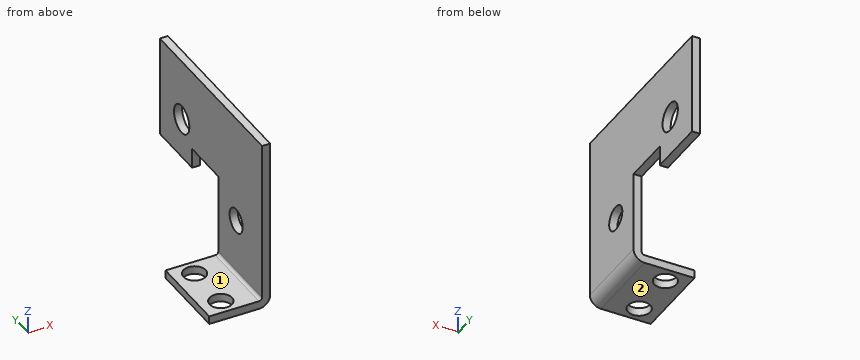
```python
from build123d import *

# Parameters (mm, degrees)
SKETCH_1_W                       = 2
SKETCH_1_H                       = 50
SM_BASE_FLANGE_1_DEPTH           = 35.2
SKETCH_7_W                       = 16.759406963
SKETCH_7_H                       = 59.520719971
CUT_EXTRUDE_2_DEPTH              = 4.8
SKETCH_9_W                       = 8.068883198
SKETCH_9_H                       = 35.697926428
CUT_EXTRUDE_3_DEPTH              = 3.23
SKETCH_6_R                       = 3.5
CUT_EXTRUDE_5_DEPTH              = 10
SKETCH_15_W                      = 15.322876818
SKETCH_15_H                      = 12
CUT_EXTRUDE_7_DEPTH              = 10
SKETCH_18_R                      = 3
CUT_EXTRUDE_8_DEPTH              = 10
SKETCH_19_W                      = 2
SKETCH_19_H                      = 14.77
SKETCH_19_H_2                    = 20
EXTRUDE_1_DEPTH                  = 2.66
SKETCH_20_W                      = 8
SKETCH_20_H                      = 14.77
CUT_EXTRUDE_9_DEPTH              = 8
SKETCH_21_W                      = 2
SKETCH_21_H                      = 20
EXTRUDE_2_DEPTH                  = 9.51
SM_EDGE_FLANGE_1_STRIP_W         = 9.4732
SM_EDGE_FLANGE_1_STRIP_H         = 2
SM_EDGE_FLANGE_1_STRIP_CUT_DEPTH = 20
SM_EDGE_FLANGE_1_DEPTH           = 20
SKETCH_27_R                      = 2.75
CUT_EXTRUDE_10_DEPTH             = 9.51


# Sheet-metal steps are written as plain solids
with BuildPart() as part:
    # Sketch 1 → 基体-法兰1 (new body)
    with BuildSketch(Plane.XY):
        with Locations((1, 25)):
            Rectangle(SKETCH_1_W, SKETCH_1_H)
    extrude(amount=SM_BASE_FLANGE_1_DEPTH)

    # 草图7 → 切除-拉伸2 (cut)
    with BuildSketch(Plane(origin=(0, 0, 0), x_dir=(-1, 0, 0), z_dir=(0, 0, -1))):
        with Locations((6.379703482, 29.760359986)):
            Rectangle(SKETCH_7_W, SKETCH_7_H)
    extrude(amount=-CUT_EXTRUDE_2_DEPTH, mode=Mode.SUBTRACT)

    # 草图9 → 切除-拉伸3 (cut)
    with BuildSketch(Plane.XZ):
        with Locations((4.034441599, 17.351036786)):
            Rectangle(SKETCH_9_W, SKETCH_9_H)
    extrude(amount=-CUT_EXTRUDE_3_DEPTH, mode=Mode.SUBTRACT)

    # 草图6 → 切除-拉伸5 (cut)
    with BuildSketch(Plane.ZY):
        with Locations((20, 40)):
            Circle(SKETCH_6_R)
    extrude(amount=-CUT_EXTRUDE_5_DEPTH, mode=Mode.SUBTRACT)

    # 草图15 → 切除-拉伸7 (cut)
    with BuildSketch(Plane.ZY):
        with Locations((7.438561591, 29.23)):
            Rectangle(SKETCH_15_W, SKETCH_15_H)
    extrude(amount=-CUT_EXTRUDE_7_DEPTH, mode=Mode.SUBTRACT)

    # 草图18 → 切除-拉伸8 (cut)
    with BuildSketch(Plane.ZY):
        with Locations((8.3960026, 15.09020987)):
            Circle(SKETCH_18_R)
    extrude(amount=-CUT_EXTRUDE_8_DEPTH, mode=Mode.SUBTRACT)

    # 草图19 → 凸台-拉伸1 (add)
    with BuildSketch(Plane(origin=(0, 0, 4.8), x_dir=(-1, 0, 0), z_dir=(0, 0, -1))):
        with Locations((-1, 42.615)):
            Rectangle(SKETCH_19_W, SKETCH_19_H)
        with Locations((-1, 13.23)):
            Rectangle(SKETCH_19_W, SKETCH_19_H_2)
    extrude(amount=EXTRUDE_1_DEPTH)

    # 草图20 → 切除-拉伸9 (cut)
    with BuildSketch(Plane.ZY):
        with Locations((6.14, 42.615)):
            Rectangle(SKETCH_20_W, SKETCH_20_H)
    extrude(amount=-CUT_EXTRUDE_9_DEPTH, mode=Mode.SUBTRACT)

    # 草图21 → 凸台-拉伸2 (add)
    with BuildSketch(Plane(origin=(0, 0, 2.14), x_dir=(-1, 0, 0), z_dir=(0, 0, -1))):
        with Locations((-1, 13.23)):
            Rectangle(SKETCH_21_W, SKETCH_21_H)
    extrude(amount=EXTRUDE_2_DEPTH)

    # 边线-法兰1 strip (across the edge) → 边线-法兰1 strip cut (cut)
    with BuildSketch(Plane(origin=(0, 23.23, -7.37), x_dir=(0, 0, 1), z_dir=(0, -1, 0))):
        with Locations((-2, -1)):
            Rectangle(SM_EDGE_FLANGE_1_STRIP_W, SM_EDGE_FLANGE_1_STRIP_H)
    extrude(amount=SM_EDGE_FLANGE_1_STRIP_CUT_DEPTH, mode=Mode.SUBTRACT)

    # 边线-法兰1 section (across the edge) → 边线-法兰1 (add)
    with BuildSketch(Plane(origin=(0, 23.23, -7.37), x_dir=(0, 0, 1), z_dir=(0, -1, 0))):
        with BuildLine():
            Line((0, 0.7366), (0, 13))
            Line((0, 13), (2, 13))
            Line((2, 13), (2, 0.7366))
            ThreePointArc((2, 0.7366), (2.215745145, 0.215745145), (2.7366, 0))
            Line((2.7366, 0), (2.7366, -2))
            ThreePointArc((2.7366, -2), (0.801531583, -1.198468417), (0, 0.7366))
        make_face()
    extrude(amount=SM_EDGE_FLANGE_1_DEPTH)

    # 草图27 → 切除-拉伸10 (cut)
    with BuildSketch(Plane.XY.offset(-5.37)):
        with Locations((-8, 19.23)):
            Circle(SKETCH_27_R)
        with Locations((-8, 7.23)):
            Circle(SKETCH_27_R)
    extrude(amount=-CUT_EXTRUDE_10_DEPTH, mode=Mode.SUBTRACT)


solid = part.part
```
Input: part model. Units: mm. Frame: model coordinates. Face numbers are marked on the shaded views. A direction names the side the tool comes from. Give positions to 0.01 mm unless a question says otherwise; leave off trailing zeros. Loops run counter-clockwise (first coordinate to the right, second up) from the corner with the lowest first, then second, coordinate; pieces in that order, holes last. Notation, with made-up numbers: (75.5, 53) -> (129.5, 53) arc R22 ccw to (129.5, 86) -> close; hole circle Ø10 at (-37, 8). An arc over 180 degrees is marked (long way). Use a Markdown table: item, result.
Q1. First-contact query: P1, Ø1.6, axis at x = 1, y = 27.5, coming from the -Z side; P2, Ø7.5, axis at x = -7, z = 7.5, coming from the +Y side; P3, Ø20, axis at y = 32, z = 15.5, coming from the -X side; P4, Ø6, axis at x = -7.5, y = 9, coming from the +Z side. Flat tips, straight axial feed; report the tip coordinate or a pass-through.
Entries:
| item | result |
|---|---|
| P1 | stops at z = 15.1 |
| P2 | passes through |
| P3 | stops at x = 0 |
| P4 | stops at z = -5.37 |
Q2. Section query D-D, the plane y = 40. Return the cut outline in (x, z).
Entries:
| item | result |
|---|---|
| outline | (0, 10.14) -> (2, 10.14) -> (2, 16.5) -> (0, 16.5) -> close; (0, 23.5) -> (2, 23.5) -> (2, 35.2) -> (0, 35.2) -> close |
Q3. Access query for the marked faces 1 and 2. Directions: +Z, -Z, +X, -X, +Y, -Y. A direction counts if a zero-diameter tool reaches every point of the face in a straight line with its end or side. Return the directions, or none.
Entries:
| item | result |
|---|---|
| face 1 | +Z, -X, +Y, -Y |
| face 2 | -Z, +X, -X, +Y, -Y |
Q4. Section query C-C, the plane x = -8. Return the cut outline in (y, z).
Entries:
| item | result |
|---|---|
| outline | (3.23, -7.37) -> (4.48, -7.37) -> (4.48, -5.37) -> (3.23, -5.37) -> close; (9.98, -7.37) -> (16.48, -7.37) -> (16.48, -5.37) -> (9.98, -5.37) -> close; (21.98, -7.37) -> (23.23, -7.37) -> (23.23, -5.37) -> (21.98, -5.37) -> close |
Q5. Section query A-A, the plane y = 7.23. Return the cut outline in (x, z), plus the area to 3 significant figures.
Entries:
| item | result |
|---|---|
| outline | (-13, -7.37) -> (-10.75, -7.37) -> (-10.75, -5.37) -> (-13, -5.37) -> close; (-5.25, -7.37) -> (-0.74, -7.37) arc R2.74 ccw to (2, -4.63) -> (2, 35.2) -> (0, 35.2) -> (0, -4.63) arc R0.74 cw to (-0.74, -5.37) -> (-5.25, -5.37) -> close |
| area | 98.6 mm² |
Q6. Section query B-B, the plane z = 20. Return the cut outline in (x, y), plus the area to 3 significant figures.
Entries:
| item | result |
|---|---|
| outline | (0, 3.23) -> (2, 3.23) -> (2, 36.5) -> (0, 36.5) -> close; (0, 43.5) -> (2, 43.5) -> (2, 50) -> (0, 50) -> close |
| area | 79.5 mm² |
Q7. Ray query, probe 1 along Y at (x, z) = (-8, -6.3); probe 2 along X at (y, z) = (29.5, 23); probe 3 along Z at (x, y) = (-11, 18). Return the intervals inside material, ascending. Write a range as from..to.
Entries:
| item | result |
|---|---|
| probe 1 | y = 3.23..4.48, 9.98..16.48, 21.98..23.23 |
| probe 2 | x = 0..2 |
| probe 3 | z = -7.37..-5.37 |
